from build123d import *

# Parameters (mm, degrees)
SKETCH_1_R               = 12.2
EXTRUDE_1_DEPTH          = 12.5
SKETCH_2_R               = 3
EXTRUDE_2_DEPTH          = 0.7
SKETCH_3_R               = 3.25
EXTRUDE_3_DEPTH          = 1
SKETCH_4_R               = 1
EXTRUDE_4_DEPTH          = 4.3
SKETCH_5_R               = 0.85
CUT_EXTRUDE_1_DEPTH      = 0.35
CUT_EXTRUDE_START        = -0.5
SKETCH_6_R               = 3.25
SKETCH_6_R_2             = 1
CUT_EXTRUDE_2_DEPTH      = 0.5
SKETCH_8_R               = 0.4
EXTRUDE_6_DEPTH          = 0.2
CUT_EXTRUDE_3_DEPTH      = 2
CUT_EXTRUDE_3_DEPTH_BACK = 1.1
SKETCH_9_R               = 0.4


with BuildPart() as part:
    # 草图1 → 凸台-拉伸1 (new body)
    with BuildSketch(Plane.XY):
        Circle(SKETCH_1_R)
    extrude(amount=EXTRUDE_1_DEPTH)

    # 草图2 → 凸台-拉伸2 (add)
    with BuildSketch(Plane.XY.offset(12.5)):
        Circle(SKETCH_2_R)
    extrude(amount=EXTRUDE_2_DEPTH)

    # 草图3 → 凸台-拉伸3 (add)
    with BuildSketch(Plane(origin=(0, 0, 0), x_dir=(-1, 0, 0), z_dir=(0, 0, -1))):
        Circle(SKETCH_3_R)
    extrude(amount=EXTRUDE_3_DEPTH)

    # 草图4 → 凸台-拉伸4 (add)
    with BuildSketch(Plane(origin=(0, 0, -1), x_dir=(-1, 0, 0), z_dir=(0, 0, -1))):
        with Locations(Location((0, 0, 0), (0, 0, 180))):
            Circle(SKETCH_4_R)
    extrude(amount=EXTRUDE_4_DEPTH)

    # 草图5 → 切除-拉伸1 (cut)
    with BuildSketch(Plane(origin=(0, 0, 0), x_dir=(-1, 0, 0), z_dir=(0, 0, -1))):
        with Locations((0, 8.25)):
            Circle(SKETCH_5_R)
        with Locations((7.144709581, 4.125)):
            Circle(SKETCH_5_R)
        with Locations((7.144709581, -4.125)):
            Circle(SKETCH_5_R)
        with Locations((0, -8.25)):
            Circle(SKETCH_5_R)
        with Locations((-7.144709581, -4.125)):
            Circle(SKETCH_5_R)
        with Locations((-7.144709581, 4.125)):
            Circle(SKETCH_5_R)
    extrude(amount=-CUT_EXTRUDE_1_DEPTH, mode=Mode.SUBTRACT)

    # 草图6 → 切除-拉伸2 (cut)
    with BuildSketch(Plane(origin=(0, 0, -1), x_dir=(-1, 0, 0), z_dir=(0, 0, -1)).offset(CUT_EXTRUDE_START)):
        Circle(SKETCH_6_R)
        with Locations(Location((0, 0, 0), (0, 0, 180))):
            Circle(SKETCH_6_R_2, mode=Mode.SUBTRACT)
    extrude(amount=CUT_EXTRUDE_2_DEPTH, mode=Mode.SUBTRACT)

    # 草图8 → 凸台-拉伸6 (add)
    # profile 1 of 2: a face of its own
    with BuildSketch(Plane(origin=(0, 0, 0), x_dir=(-1, 0, 0), z_dir=(0, 0, -1))):
        with BuildLine():
            Line((0.694469448, 12.85), (0.694469448, 12.180218068))
            add(Edge.make_bspline(
                [(0.694469448, 12.180218068), (0, 12.219781932), (-0.694469448, 12.180218068)],
                knots=[0, 0, 0, 1, 1, 1], degree=2))
            Line((-0.694469448, 12.180218068), (-0.694469448, 12.85))
            add(Edge.make_bspline(
                [(0.694469448, 12.85), (0, 14.15), (-0.694469448, 12.85)],
                knots=[0, 0, 0, 1, 1, 1], degree=2))
        make_face()
        with Locations((0, 12.85)):
            Circle(SKETCH_8_R, mode=Mode.SUBTRACT)
    # profile 2 of 2: a face of its own
    with BuildSketch(Plane(origin=(0, 0, 0), x_dir=(-1, 0, 0), z_dir=(0, 0, -1))):
        with BuildLine():
            Line((-0.694469448, -12.85), (-0.694469448, -12.180218068))
            add(Edge.make_bspline(
                [(0.694469448, -12.180218068), (0, -12.219781932), (-0.694469448, -12.180218068)],
                knots=[0, 0, 0, 1, 1, 1], degree=2))
            Line((0.694469448, -12.180218068), (0.694469448, -12.85))
            add(Edge.make_bspline(
                [(0.694469448, -12.85), (0, -14.15), (-0.694469448, -12.85)],
                knots=[0, 0, 0, 1, 1, 1], degree=2))
        make_face()
        with Locations((0, -12.85)):
            Circle(SKETCH_8_R, mode=Mode.SUBTRACT)
    extrude(amount=-EXTRUDE_6_DEPTH)

    # 草图9 → 切除-拉伸3 (cut, two sides: drawn at the far end of the back side and taken through both)
    with BuildSketch(Plane(origin=(-65.68529626, 3.340628685, 41.676272609), x_dir=(0, 0, -1), z_dir=(0.08103812035682426, 0.9967110027731373, 1.0147062402532315e-14)).offset(-CUT_EXTRUDE_3_DEPTH_BACK)):
        with Locations(Location((43.872176256, -65.74, 0), (0, 0, 270))):
            Circle(SKETCH_9_R)
    extrude(amount=CUT_EXTRUDE_3_DEPTH + CUT_EXTRUDE_3_DEPTH_BACK, mode=Mode.SUBTRACT)


solid = part.part
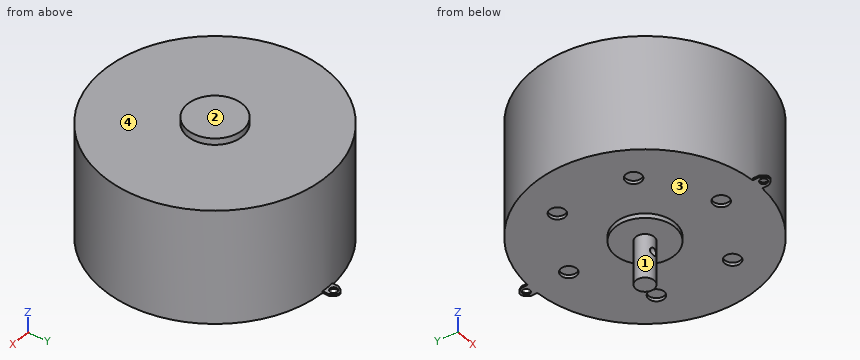
Verification items for the finished model (mm, model axes). Face numbers are marked on the shaded views. A direction names the side the tool comes from. Coordinates: 2 decimals unless noted, no trailing zeros. Loops run counter-clockwise (first coordinate to the right, second up) from the corner with the lowest first, then second, coordinate; pieces in that order, holes last. Notation, with made-up numbers: (-30.75, 66) -> (7.25, 66) arc R10 ccw to (7.25, 72) -> close; hole circle Ø7 at (25.25, -2). An arc over 180 degrees is marked (long way). Answer as CSV lines item,"result".
1) Thickness scan on L1, parallel to Y at x = 0, z = 0.1; L2, parallel to Z at x = -3.25, y = 11.5; L3, parallel to Z at x = 1, y = 2.75. Record the ranges inside material, lowest first. Write a range as from..to.
Found:
L1,"y = -13.5..-13.25, -12.45..-9.1, -7.4..7.4, 9.1..12.45, 13.25..13.5"
L2,"z = 0..12.5"
L3,"z = -0.5..13.2"
2) Release check for a two-part mould opening along Y. For the marked faces 1 and 2 record: +Y half, -Y half, draft (parallel to the pull), parting line (faces both ways), or undercut.
Found:
face 1,"parting line"
face 2,"draft"
3) Cross-section at D-D, the plane y = 8.25. Record the cut outline in (x, z), then the cut area to 3 significant figures.
Found:
outline,"(-8.99, 0) -> (-0.85, 0) -> (-0.85, 0.35) -> (0.85, 0.35) -> (0.85, 0) -> (8.99, 0) -> (8.99, 12.5) -> (-8.99, 12.5) -> close"
area,"224 mm2"
4) Cross-section at C-C, the plane z = 8. Record the cut outline in (x, y), then the cut area to 3 significant figures.
Found:
outline,"circle Ø24.4 at (0, 0)"
area,"468 mm2"
5) Tool access check on the marked faces 3 and 4. Record the directions out of +Z, -Z, +X, -X, +Y, -Y that give a thin tool (end or side, any length) a straight path to the whole face; none if there is none.
Found:
face 3,"-Z"
face 4,"+Z"
6) Cross-section at B-B, the plane x = -2.25. Record the cut outline in (y, z).
Found:
outline,"(-11.99, 0) -> (-2.35, 0) -> (-2.35, -0.5) -> (2.35, -0.5) -> (2.35, 0) -> (11.99, 0) -> (11.99, 12.5) -> (1.98, 12.5) -> (1.98, 13.2) -> (-1.98, 13.2) -> (-1.98, 12.5) -> (-11.99, 12.5) -> close"
7) Cross-section at A-A, the plane y = 1.75. Record the cut outline in (x, z), then the cut area to 3 significant figures.
Found:
outline,"(-12.07, 0) -> (-2.74, 0) -> (-2.74, -0.5) -> (2.74, -0.5) -> (2.74, 0) -> (12.07, 0) -> (12.07, 12.5) -> (2.44, 12.5) -> (2.44, 13.2) -> (-2.44, 13.2) -> (-2.44, 12.5) -> (-12.07, 12.5) -> close"
area,"308 mm2"
8) Depth check by flat-ended pin: pin 1 (6 mm diameter, centred on x = -0.5, z = 11, fed in from -Y); pin 2 (1.4 mm diameter, centred on x = 7, y = -4, fed in from -Z); pin 3 (6 mm diameter, centred on x = 8.5, z = 1, fed in from -Y). Enter the tip coordinate at first touch or a pass-through.
Found:
pin 1,"stops at y = -12.2"
pin 2,"stops at z = 0"
pin 3,"stops at y = -10.89"
